Read the model definition and answer for the solid it produces. Units are mm, in the model's axes. A direction names the side the tool comes from. Coordinates: 2 decimals unless noted, no trailing zeros. Loops run counter-clockwise (first coordinate to the right, second up) from the corner with the lowest first, then second, coordinate; pieces in that order, holes last. Notation, with made-up numbers: (6, 73) - (26, 73) arc R14 cw to (26, 86) - close; hole circle Ø9 at (5, 21.5). An arc over 180 degrees is marked (long way). One line per item, written item: value. Start each with the question number.
from build123d import *

# Parameters (mm, degrees)
BOSS_EXTRUDE1_DEPTH = 60
FILLET1_R           = 5
SHELL1_T            = -2
SKETCH2_R           = 2.675
BOSS_EXTRUDE2_DEPTH = 27
SKETCH3_R           = 1.425
CUT_EXTRUDE1_DEPTH  = 4
SKETCH4_W           = 18
SKETCH4_H           = 3
BOSS_EXTRUDE3_DEPTH = 88
SKETCH5_R           = 2
CUT_EXTRUDE2_DEPTH  = 3
BOSS_EXTRUDE4_DEPTH = 88
SKETCH8_R           = 1.5
CUT_EXTRUDE3_DEPTH  = 2
SKETCH9_R           = 2.5
BOSS_EXTRUDE5_DEPTH = 1
SKETCH10_R          = 4
SKETCH10_R_2        = 1.5
SKETCH10_R_3        = 2
CUT_EXTRUDE4_DEPTH  = 1
SKETCH11_R          = 2.425
SKETCH11_R_2        = 1.425
BOSS_EXTRUDE6_DEPTH = 3


with BuildPart() as part:
    # Sketch1 → Boss-Extrude1 (new body)
    with BuildSketch(Plane(origin=(0, 0, 0), x_dir=(0, 0, -1), z_dir=(1, 0, 0))):
        with BuildLine():
            Line((35, 0), (118, 0))
            Line((118, 0), (118, 90))
            Line((118, 90), (-82, 90))
            Line((-82, 90), (-82, 0))
            Line((-82, 0), (-35, 0))
            ThreePointArc((-35, 0), (0, 35), (35, 0))
        make_face()
    extrude(amount=BOSS_EXTRUDE1_DEPTH)

    # Fillet1
    fillet1_edges = [part.edges().sort_by_distance(p)[0] for p in [
        (60, 45, -118),
        (30, 90, -118),
        (60, 90, -18),
    ]]
    fillet(fillet1_edges, radius=FILLET1_R)

    # Shell1
    shell1_openings = [part.faces().sort_by_distance(p)[0] for p in [
        (30, 0, 58.5),
        (29.971275261, 44.956357534, 82),
        (29.96885008, 0, -76.456447556),
        (30, 17.5, 0),
        (0, 48.594891541, -20.122257458),
    ]]
    offset(amount=SHELL1_T, openings=shell1_openings, kind=Kind.INTERSECTION)

    # Sketch2 → Boss-Extrude2 (add)
    with BuildSketch(Plane.XZ.offset(-88)):
        with Locations(Location((41, -76, 0), (0, 0, 270))):  # turned: the seam where the file's is
            Circle(SKETCH2_R)
    extrude(amount=BOSS_EXTRUDE2_DEPTH)

    # Sketch3 → Cut-Extrude1 (cut)
    with BuildSketch(Plane.XZ.offset(-61)):
        with Locations(Location((41, -76, 0), (0, 0, 270))):  # turned: the seam where the file's is
            Circle(SKETCH3_R)
    extrude(amount=-CUT_EXTRUDE1_DEPTH, mode=Mode.SUBTRACT)

    # Sketch4 → Boss-Extrude3 (add)
    with BuildSketch(Plane.XZ):
        with Locations((49, 80.5)):
            Rectangle(SKETCH4_W, SKETCH4_H)
    extrude(amount=-BOSS_EXTRUDE3_DEPTH)

    # Sketch5 → Cut-Extrude2 (cut)
    with BuildSketch(Plane.XY.offset(82)):
        with Locations((50, 25)):
            Circle(SKETCH5_R)
        with Locations((50, 65)):
            Circle(SKETCH5_R)
    extrude(amount=-CUT_EXTRUDE2_DEPTH, mode=Mode.SUBTRACT)

    # Sketch6 → Boss-Extrude4 (add)
    with BuildSketch(Plane.XZ):
        Polygon((58, 35), (35, 35), (35, 12.5), (15, 12.5), (15, -12.5), (35, -12.5), (35, -35), (58, -35), (58, -36), (34, -36), (34, -13.5), (14, -13.5), (14, 13.5), (34, 13.5), (34, 36), (58, 36), align=None)
    extrude(amount=-BOSS_EXTRUDE4_DEPTH)

    # Sketch8 → Cut-Extrude3 (cut)
    with BuildSketch(Plane(origin=(0, 90, 0), x_dir=(1, 0, 0), z_dir=(0, 1, 0))):
        with Locations(Location((48, 106, 0), (0, 0, 270))):  # turned: the seam where the file's is
            Circle(SKETCH8_R)
    extrude(amount=-CUT_EXTRUDE3_DEPTH, mode=Mode.SUBTRACT)

    # Sketch9 → Boss-Extrude5 (add)
    with BuildSketch(Plane.XZ.offset(-88)):
        with Locations(Location((48, -106, 0), (0, 0, 270))):  # turned: the seam where the file's is
            Circle(SKETCH9_R)
        with BuildLine():
            Line((46.585786438, -105.5), (49.414213562, -105.5))
            ThreePointArc((49.414213562, -105.5), (49.5, -106), (49.414213562, -106.5))
            Line((49.414213562, -106.5), (46.585786438, -106.5))
            ThreePointArc((46.585786438, -106.5), (46.5, -106), (46.585786438, -105.5))
        make_face(mode=Mode.SUBTRACT)
    extrude(amount=BOSS_EXTRUDE5_DEPTH)

    # Sketch10 → Cut-Extrude4 (cut)
    with BuildSketch(Plane.ZY.offset(-14)):
        Circle(SKETCH10_R)
        with Locations((-8.75, 20.5)):
            Circle(SKETCH10_R_2)
        with Locations((8.75, 20.5)):
            Circle(SKETCH10_R_2)
        with Locations((-8.75, 47)):
            Circle(SKETCH10_R_3)
        with Locations((8.75, 47)):
            Circle(SKETCH10_R_3)
    extrude(amount=-CUT_EXTRUDE4_DEPTH, mode=Mode.SUBTRACT)

    # Mirror1: part across plane


with BuildPart() as part_1:
    add(part.part)
    add(part.part.mirror(Plane(origin=(0, 0, 0), x_dir=(0, 0, 1), z_dir=(1, 0, 0))))

    # Sketch11 → Boss-Extrude6 (add)
    with BuildSketch(Plane.XZ.offset(-88)):
        with Locations(Location((18.69, 23.5, 0), (0, 0, 270))):  # turned: the seam where the file's is
            Circle(SKETCH11_R)
        with Locations(Location((18.69, 23.5, 0), (0, 0, 270))):  # turned: the seam where the file's is
            Circle(SKETCH11_R_2, mode=Mode.SUBTRACT)
        with Locations(Location((18.69, 60.24, 0), (0, 0, 270))):  # turned: the seam where the file's is
            Circle(SKETCH11_R)
        with Locations(Location((18.69, 60.24, 0), (0, 0, 270))):  # turned: the seam where the file's is
            Circle(SKETCH11_R_2, mode=Mode.SUBTRACT)
        with Locations(Location((-18.69, 60.24, 0), (0, 0, 270))):  # turned: the seam where the file's is
            Circle(SKETCH11_R)
        with Locations(Location((-18.69, 60.24, 0), (0, 0, 270))):  # turned: the seam where the file's is
            Circle(SKETCH11_R_2, mode=Mode.SUBTRACT)
        with Locations(Location((-18.69, 23.5, 0), (0, 0, 270))):  # turned: the seam where the file's is
            Circle(SKETCH11_R)
        with Locations(Location((-18.69, 23.5, 0), (0, 0, 270))):  # turned: the seam where the file's is
            Circle(SKETCH11_R_2, mode=Mode.SUBTRACT)
    extrude(amount=BOSS_EXTRUDE6_DEPTH)


solid = part_1.part
1) Section A-A, the plane z = 45 is taken. Determine the outline of the cut face in (x, y).
2) For faces 4 (the cylindrical face through (-51.075, 66.686, 80.521)), 5 (the flat face through (-20, 85, 59)), 6 (the cylindrical face through (-14.493, 45.048, -9.184)), 7 (the flat face through (58, 43, 58)), 8 (the flat face through (1, 42, -118)), determine the directions among +Z, -Z, +X, -X, +Y, -Y from which every point of the face is accessible in a straight line to the end or side of a thin tool.
3) Flat-ended cylindrical pins translate along their axes: P1, Ø12, axis at x = -25.5, z = -59.5, coming from the -Y side; P2, Ø1.5, axis at x = -48, z = -105.5, coming from the -Y side; P3, Ø1.4, axis at x = -18.5, z = 59.5, coming from the -Y side. Find the tip coordinate at first contact, or state that the pin passes through.
4) Straight lines are drawn through the part: L1, parallel to Z at x = 44.5, y = 68.5; L2, parallel to Z at x = 25, y = 53.5; L3, parallel to X at y = 44, z = -7. For each, find the intervals that lie inside material, in ascending order.
5) Determine the mould class of faces 1 (the flat face through (40.3, 51.5, 82)), 2 (the cylindrical face through (-1, 88, -117)), 3 (the cylindrical face through (14.493, 45.048, 8.316)) for opening direction Y: released by +Y, released by -Y, zero draft, split by the parting line, or undercut.
6) Section C-C, the plane x = 29.5 is taken. Determine the outline of the cut face in (y, z), and give its area (3 significant figures).
7) Section B-B, the plane y = 69 is taken. State how many separate pieces and enclosed holes the cut face has, and give its area (3 significant figures).
Answer below:
1. outline: (-60, 0) - (-58, 0) - (-58, 85) arc R3 cw to (-55, 88) - (55, 88) arc R3 cw to (58, 85) - (58, 0) - (60, 0) - (60, 85) arc R5 ccw to (55, 90) - (-55, 90) arc R5 ccw to (-60, 85) - close
2. face 4: +Z
2. face 5: +Z, -Y
2. face 6: none
2. face 7: -Y
2. face 8: -Z, +X, -X, +Y, -Y
3. P1: y = 88
3. P2: y = 87
3. P3: y = 85
4. L1: -118 to -116, -36 to -35, 35 to 36, 79 to 82
4. L2: -118 to -116, -13.5 to -12.5, 12.5 to 13.5
4. L3: -60 to -58, -15 to -14, 14 to 15, 58 to 60
5. face 1: zero draft
5. face 2: released by +Y
5. face 3: undercut
6. outline: (0, -118) - (85, -118) arc R5 ccw to (90, -113) - (90, 82) - (88, 82) - (88, 13.5) - (0, 13.5) - (0, 12.5) - (88, 12.5) - (88, -12.5) - (0, -12.5) - (0, -13.5) - (88, -13.5) - (88, -113) arc R3 cw to (85, -116) - (0, -116) - close
6. area: 749 mm2
7. separate pieces: 3
7. enclosed holes: 2
7. area: 1,490 mm2
